```python
from build123d import *

# Parameters (mm, degrees)
BOSS_EXTRUDE1_DEPTH  = 3.5
SKETCH3_W            = 35
SKETCH3_H            = 40
BOSS_EXTRUDE2_DEPTH  = 17
SKETCH5_W            = 32.32
SKETCH5_H            = 12.1
CUT_EXTRUDE1_DEPTH   = 10.75
SKETCH6_W            = 28.5
SKETCH6_H            = 12.5
CUT_EXTRUDE2_DEPTH   = 17
SKETCH10_R           = 3
BOSS_EXTRUDE7_DEPTH  = 5
SKETCH11_R           = 3
BOSS_EXTRUDE8_DEPTH  = 5
SKETCH12_W           = 9
SKETCH12_H           = 6.5
CUT_EXTRUDE3_DEPTH   = 20
SKETCH13_W           = 17
SKETCH13_H           = 6.985272442
CUT_EXTRUDE4_DEPTH   = 140.119509628
SKETCH14_W           = 17
SKETCH14_H           = 3.182225524
CUT_EXTRUDE5_DEPTH   = 140.119509628
SKETCH15_W           = 13.15864123
SKETCH15_H           = 11.411738648
SKETCH15_W_2         = 10.578454188
SKETCH15_H_2         = 8.248928726
BOSS_EXTRUDE9_DEPTH  = 75
SKETCH16_W           = 1.920679385
SKETCH16_H           = 11.453083587
BOSS_EXTRUDE10_DEPTH = 75


with BuildPart() as part:
    # Sketch2 → Boss-Extrude1 (new body)
    with BuildSketch(Plane.XY):
        with BuildLine():
            Line((65, -99.543899658), (-65, -99.543899658))
            ThreePointArc((-65, -99.543899658), (-72.071067812, -96.61496747), (-75, -89.543899658))
            Line((-75, -89.543899658), (-75, 40.456100342))
            ThreePointArc((-75, 40.456100342), (-72.071067812, 47.527168154), (-65, 50.456100342))
            Line((-65, 50.456100342), (65, 50.456100342))
            ThreePointArc((65, 50.456100342), (72.071067812, 47.527168154), (75, 40.456100342))
            Line((75, 40.456100342), (75, -89.543899658))
            ThreePointArc((75, -89.543899658), (72.071067812, -96.61496747), (65, -99.543899658))
        make_face()
    extrude(amount=BOSS_EXTRUDE1_DEPTH)

    # Sketch3 → Boss-Extrude2 (add)
    with BuildSketch(Plane.XY.offset(3.5)):
        with Locations((37.5, -64.543899658)):
            Rectangle(SKETCH3_W, SKETCH3_H)
    extrude(amount=BOSS_EXTRUDE2_DEPTH)

    # Sketch5 → Cut-Extrude1 (cut)
    with BuildSketch(Plane.XZ.offset(84.543899658)):
        with Locations((37.5, 12)):
            Rectangle(SKETCH5_W, SKETCH5_H)
    extrude(amount=-CUT_EXTRUDE1_DEPTH, mode=Mode.SUBTRACT)

    # Sketch6 → Cut-Extrude2 (cut)
    with BuildSketch(Plane.XZ.offset(73.793899658)):
        with Locations((37.5, 12)):
            Rectangle(SKETCH6_W, SKETCH6_H)
    extrude(amount=-CUT_EXTRUDE2_DEPTH, mode=Mode.SUBTRACT)

    # Sketch10 → Boss-Extrude7 (add)
    with BuildSketch(Plane.XY.offset(3.5)):
        with Locations(Location((0, -92.043899658, 0), (0, 0, 180))):
            Circle(SKETCH10_R)
        with Locations(Location((-66, -92.043899658, 0), (0, 0, 180))):
            Circle(SKETCH10_R)
    extrude(amount=BOSS_EXTRUDE7_DEPTH)

    # Sketch11 → Boss-Extrude8 (add)
    with BuildSketch(Plane.XY.offset(3.5)):
        with Locations(Location((-66, 42.956100342, 0), (0, 0, 180))):
            Circle(SKETCH11_R)
        with Locations(Location((66, 42.956100342, 0), (0, 0, 180))):
            Circle(SKETCH11_R)
    extrude(amount=BOSS_EXTRUDE8_DEPTH)

    # Sketch12 → Cut-Extrude3 (cut)
    with BuildSketch(Plane.ZY.offset(-20)):
        with Locations((12, -61.493899658)):
            Rectangle(SKETCH12_W, SKETCH12_H)
    extrude(amount=-CUT_EXTRUDE3_DEPTH, mode=Mode.SUBTRACT)

    # Sketch13 → Cut-Extrude4 (cut, through all)
    with BuildSketch(Plane.ZY.offset(-20)):
        with Locations((12, -48.036535879)):
            Rectangle(SKETCH13_W, SKETCH13_H)
    extrude(amount=-CUT_EXTRUDE4_DEPTH, mode=Mode.SUBTRACT)

    # Sketch14 → Cut-Extrude5 (cut, through all)
    with BuildSketch(Plane.ZY.offset(-20)):
        with Locations((12, -53.120284862)):
            Rectangle(SKETCH14_W, SKETCH14_H)
    extrude(amount=-CUT_EXTRUDE5_DEPTH, mode=Mode.SUBTRACT)

    # Sketch15 → Boss-Extrude9 (add)
    with BuildSketch(Plane.ZY.offset(-20)):
        with Locations((12, -61.493899658)):
            Rectangle(SKETCH15_W, SKETCH15_H)
        with Locations((12, -61.493899658)):
            Rectangle(SKETCH15_W_2, SKETCH15_H_2, mode=Mode.SUBTRACT)
    extrude(amount=BOSS_EXTRUDE9_DEPTH)

    # Sketch16 → Boss-Extrude10 (add)
    with BuildSketch(Plane.ZY.offset(-20)):
        with Locations((4.460339692, -61.514572128)):
            Rectangle(SKETCH16_W, SKETCH16_H)
    extrude(amount=BOSS_EXTRUDE10_DEPTH)


solid = part.part
```
Could you check a few things on this model? Use its own coordinates, in mm. A direction names the side the tool comes from. Round coordinates to 2 decimals unless told otherwise and drop trailing zeros. Loops run counter-clockwise (first coordinate to the right, second up) from the corner with the lowest first, then second, coordinate; pieces in that order, holes last.
Q1. I want a section at C-C (x = 45.5). Write out the boundary of the cut face in (y, z), and give its area (3 significant figures).
Q2. Thinking about a two-plate mould opening in Y: for faces 4 (the flat face through (-1, 50.456, 2)), 5 (the flat face through (37, -65, 18.25)), 6 (the flat face through (-75, -25, 2)), which applies, pulls with the +Y half, pulls with the -Y half, needs draft (parallel to the pull), parting line crosses it, or undercut?
Q3. For P1, Ø12.5, axis at x = -26, y = -62.5, coming from the +Z side; P2, Ø2, axis at x = 53, z = 13.5, coming from the -Y side; P3, Ø12, axis at y = -81, z = 10, coming from the -X side; P4, Ø18.5, axis at x = 43, y = -68.5, coming from the -Z side, each with a flat end and sliding along its axis, tell me the tip position at first contact or that it passes through.
Q4. I want a section at B-B (y = -76). Write out the boundary of the cut face in (x, z).
Q5. On a 3-axis mill with a long thin cutter (end or side, diameter ignored), from which of +Z, -Z, +X, -X, +Y, -Y can I reach the whole of each face in a straight line? I mean faces 1 (the flat face through (53.66, -79, 12)), 2 (the cylindrical face through (0.65, -89.115, 5.965)), 3 (the flat face through (-17, -65.618, 12)). Say none if no direction works.
Q6. I want a section at A-A (x = 0). Write out the boundary of the cut face in (y, z), and give its area (3 significant figures).
Q7. I want a section at D-D (y = -33.5). Write out the boundary of the cut face in (x, z), and give its area (3 significant figures).
Q8. Please list where these lines run through material, in increasing order: L1, parallel to X at y = -82, z = 13; L2, parallel to Y at x = -49, z = 15.25; L3, parallel to Y at x = -1, z = 7.
Answer below:
1. outline: (-99.54, 0) - (50.46, 0) - (50.46, 3.5) - (-54.71, 3.5) - (-54.71, 20.5) - (-84.54, 20.5) - (-84.54, 18.05) - (-73.79, 18.05) - (-73.79, 18.25) - (-56.79, 18.25) - (-56.79, 5.75) - (-73.79, 5.75) - (-73.79, 5.95) - (-84.54, 5.95) - (-84.54, 3.5) - (-99.54, 3.5) - close
1. area: 690 mm2
2. face 4: pulls with the +Y half
2. face 5: undercut
2. face 6: needs draft
3. P1: stops at z = 18.58
3. P2: stops at y = -84.54
3. P3: stops at x = 20
3. P4: stops at z = 0
4. outline: (-75, 0) - (75, 0) - (75, 3.5) - (55, 3.5) - (55, 20.5) - (20, 20.5) - (20, 3.5) - (-75, 3.5) - close; hole (21.34, 5.95) - (53.66, 5.95) - (53.66, 18.05) - (21.34, 18.05) - close
5. face 1: -Y
5. face 2: +Z
5. face 3: -X
6. outline: (-99.54, 0) - (50.46, 0) - (50.46, 3.5) - (-55.79, 3.5) - (-55.79, 18.58) - (-67.2, 18.58) - (-67.2, 5.42) - (-67.24, 5.42) - (-67.24, 3.5) - (-89.04, 3.5) - (-89.04, 8.5) - (-95.04, 8.5) - (-95.04, 3.5) - (-99.54, 3.5) - close; hole (-65.62, 6.71) - (-57.37, 6.71) - (-57.37, 17.29) - (-65.62, 17.29) - close
6. area: 640 mm2
7. outline: (-75, 0) - (75, 0) - (75, 3.5) - (-75, 3.5) - close
7. area: 525 mm2
8. L1: x = 20 to 21.34, 53.66 to 55
8. L2: y = -67.2 to -65.62, -57.37 to -55.79
8. L3: y = -94.87 to -89.22, -67.2 to -65.62, -57.37 to -55.79
